Print and shaded views of the part. All mm, measured from the part's lowest x, y and z. A direction names the side the tool comes from. Coordinates: 2 decimals unless noted, no trailing zeros. Order: outer loops, then holes, each group sorted by start corner. A loop starts at its lowest first (then second) coordinate and runs counter-clockwise, first axis right, second up. Notation, with made-up numbers: (47.25, -35) -> (55.25, -35) arc R25 cw to (55.25, 2) -> close; hole circle Ø1 at (-39.5, 67). An arc over 180 degrees is marked (long way). Return JSON: item names as keys, results as strings. Group by question number.
1) Which spindle directions (+Z, -Z, +X, -X, +Y, -Y) get a long thin tool onto all of the face, cutting with end or side? Do the marked faces 1, 2 and 3. Say none if no direction does.
2) Cut at A-A (y = 3). Write the cut outline in (x, z).
3) Cut at D-D (y = 12). Write the cut outline in (x, z).
4) Cut at C-C (x = 14.5). Write the cut outline in (y, z).
5) Probe line 1 (X direction, y = 15, z = 14); line 2 (Z direction, x = 5.5, y = 29.5); line 3 (Y direction, x = 7, z = 25). List the from-to ranges inside material, lowest first.
6) Cut at B-B (z = 37). Write the cut outline in (x, y), and give its area (3 significant figures).
7) Flat gauge pins, fed straight in: pin 1 (14 mm diameter, centred on x = 29.5, y = 12, fed in from -Z); pin 2 (5.5 mm diameter, centred on y = 28, z = 11, fed in from +X); pin 3 (6.5 mm diameter, centred on x = 6.5, y = 27.5, fed in from -Z); pin 4 (6 mm diameter, centred on x = 33.5, z = 18, fed in from -Y). Where does each tip first touch, or does it go through?
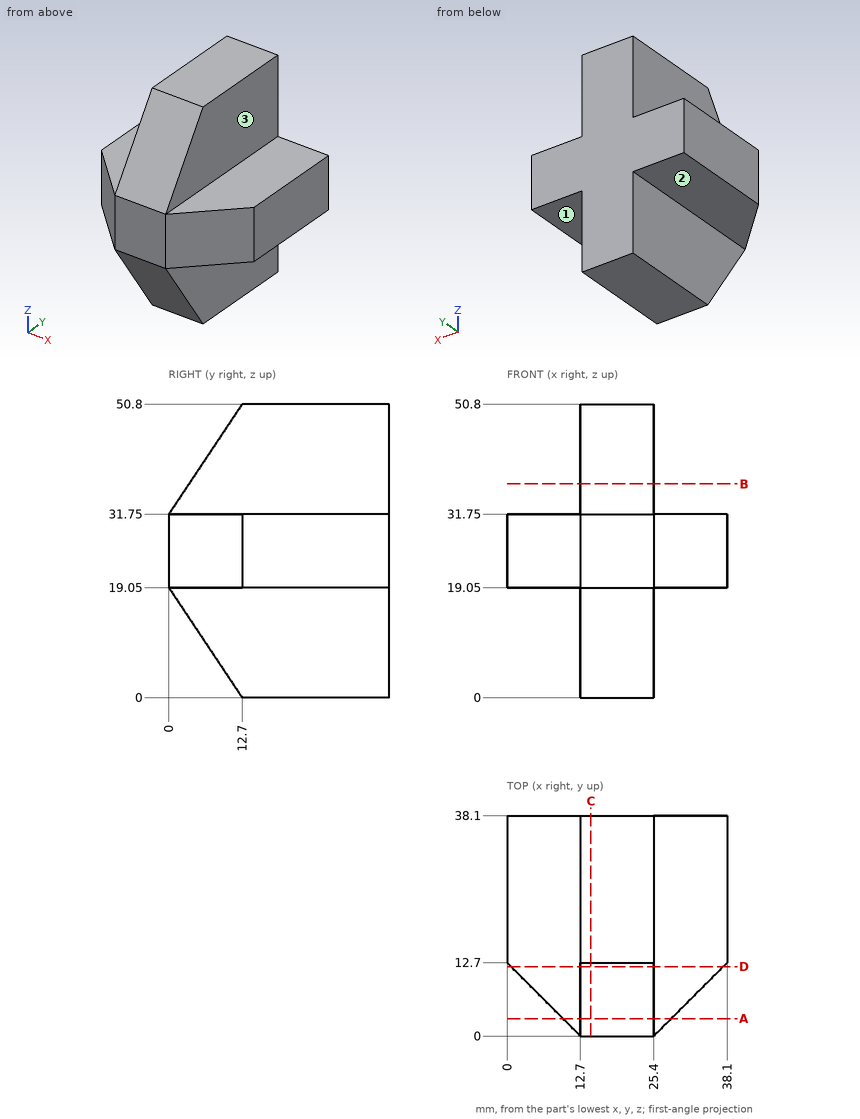
Answers below:
{
 "1": {"face 1": "-Z, +X, +Y, -Y", "face 2": "-Z, -X, +Y, -Y", "face 3": "+Z, +X, +Y, -Y"},
 "2": {"outline": "(9.7, 19.05) -> (12.7, 19.05) -> (12.7, 14.55) -> (25.4, 14.55) -> (25.4, 19.05) -> (28.4, 19.05) -> (28.4, 31.75) -> (25.4, 31.75) -> (25.4, 36.25) -> (12.7, 36.25) -> (12.7, 31.75) -> (9.7, 31.75) -> close"},
 "3": {"outline": "(0.7, 19.05) -> (12.7, 19.05) -> (12.7, 1.05) -> (25.4, 1.05) -> (25.4, 19.05) -> (37.4, 19.05) -> (37.4, 31.75) -> (25.4, 31.75) -> (25.4, 49.75) -> (12.7, 49.75) -> (12.7, 31.75) -> (0.7, 31.75) -> close"},
 "4": {"outline": "(0, 19.05) -> (12.7, 0) -> (38.1, 0) -> (38.1, 50.8) -> (12.7, 50.8) -> (0, 31.75) -> close"},
 "5": {"line 1": "x = 12.7 to 25.4", "line 2": "z = 19.05 to 31.75", "line 3": "y = 5.7 to 38.1"},
 "6": {"outline": "(12.7, 3.5) -> (25.4, 3.5) -> (25.4, 38.1) -> (12.7, 38.1) -> close", "area": "439 mm^2"},
 "7": {"pin 1": "stops at z = 0", "pin 2": "stops at x = 25.4", "pin 3": "stops at z = 19.05", "pin 4": "stops at y = 5.29"}
}
